Source: CAD feature listing. Evaluate the final solid. Frame: model axes, mm. A direction names the side the tool comes from. Give positions to 0.01 mm unless a question says otherwise; leave off trailing zeros. Order: outer loops, then holes, each group sorted by start corner. A loop starts at its lowest first (then second) coordinate and runs counter-clockwise, first axis right, second up.
from build123d import *

# Parameters (mm, degrees)
SKETCH_W      = 15.4
SKETCH_H      = 61
PAD_DEPTH     = 3
FILLET_R      = 4
PAD001_DEPTH  = 5
PAD002_DEPTH  = 5
SKETCH003_W   = 15.4
SKETCH003_H   = 6
PAD003_DEPTH  = 49
FILLET001_R   = 2.2
FILLET002_R   = 20
FILLET003_R   = 2.2
SKETCH004_W   = 4
SKETCH004_H   = 17
SKETCH004_W_2 = 2
SKETCH004_H_2 = 11
SKETCH004_W_3 = 2.5
SKETCH004_H_3 = 21
POCKET_DEPTH  = 54.801


with BuildPart() as part:
    # Sketch → Pad (new body)
    with BuildSketch(Plane.XZ):
        Rectangle(SKETCH_W, SKETCH_H)
    extrude(amount=PAD_DEPTH)

    # Fillet
    fillet_edges = [part.edges().sort_by_distance(p)[0] for p in [
        (7.7, -1.5, 30.5),
        (-7.7, -1.5, 30.5),
        (7.7, -1.5, -30.5),
        (-7.7, -1.5, -30.5),
    ]]
    fillet(fillet_edges, radius=FILLET_R)

    # Sketch001 (on Face2 of Fillet) → Pad001 (join)
    with BuildSketch(Plane(origin=(0, 0, 0), x_dir=(1, 0, 0), z_dir=(0, 1, 0))):
        with BuildLine():
            Line((-2.2, 16.65), (-2.2, 14.55))
            ThreePointArc((-2.2, 14.55), (0, 12.35), (2.2, 14.55))
            Line((2.2, 16.65), (2.2, 14.55))
            ThreePointArc((2.2, 16.65), (0, 18.85), (-2.2, 16.65))
        make_face()
        with BuildLine():
            Line((-2.2, -14.55), (-2.2, -16.65))
            ThreePointArc((-2.2, -16.65), (0, -18.85), (2.2, -16.65))
            Line((2.2, -14.55), (2.2, -16.65))
            ThreePointArc((2.2, -14.55), (0, -12.35), (-2.2, -14.55))
        make_face()
    extrude(amount=PAD001_DEPTH)

    # Sketch002 (on Face19 of Pad001) → Pad002 (join)
    with BuildSketch(Plane(origin=(0, 5, 0), x_dir=(1, 0, 0), z_dir=(0, 1, 0))):
        with BuildLine():
            Line((-2.2, 23.15), (-2.2, 14.55))
            ThreePointArc((-2.2, 14.55), (0, 12.35), (2.2, 14.55))
            Line((2.2, 23.15), (2.2, 14.55))
            ThreePointArc((2.2, 23.15), (0, 25.35), (-2.2, 23.15))
        make_face()
        with BuildLine():
            Line((-2.2, -8.05), (-2.2, -16.65))
            ThreePointArc((-2.2, -16.65), (0, -18.85), (2.2, -16.65))
            Line((2.2, -8.05), (2.2, -16.65))
            ThreePointArc((2.2, -8.05), (0, -5.85), (-2.2, -8.05))
        make_face()
    extrude(amount=PAD002_DEPTH)

    # Sketch003 (on Face5 of Pad002) → Pad003 (join)
    with BuildSketch(Plane.XZ.offset(3)):
        with Locations((0, 21.3)):
            Rectangle(SKETCH003_W, SKETCH003_H)
    extrude(amount=PAD003_DEPTH)

    # Fillet001
    fillet001_edges = [part.edges().sort_by_distance(p)[0] for p in [
        (7.7, -52, 21.3),
        (-7.7, -52, 21.3),
    ]]
    fillet(fillet001_edges, radius=FILLET001_R)

    # Fillet002
    fillet002_edges = [part.edges().sort_by_distance(p)[0] for p in [
        (0, -3, 18.3),
    ]]
    fillet(fillet002_edges, radius=FILLET002_R)

    # Fillet003
    fillet003_edges = [part.edges().sort_by_distance(p)[0] for p in [
        (0, -3, 24.3),
    ]]
    fillet(fillet003_edges, radius=FILLET003_R)

    # Sketch004 (on Face2 of Fillet003) → Pocket (cut, through all)
    with BuildSketch(Plane(origin=(0, 0, 24.3), x_dir=(-1, 0, 0), z_dir=(0, 0, 1))):
        with Locations((2.7, 15.5)):
            Rectangle(SKETCH004_W, SKETCH004_H)
        with Locations((2.7, 36.5)):
            Rectangle(SKETCH004_W_2, SKETCH004_H_2)
        with Locations((-3.55, 24.5)):
            Rectangle(SKETCH004_W_3, SKETCH004_H_3)
    extrude(amount=-POCKET_DEPTH, mode=Mode.SUBTRACT)


solid = part.part
1) Section query B-B on z = 11.5. Output: boundary loops of the cut face in (x, y).
Checks:
outline: (-7.7, -7.97) - (-4.7, -7.97) - (-4.7, -7) - (-0.7, -7) - (-0.7, -7.97) - (7.7, -7.97) - (7.7, 0) - (-7.7, 0) - close; (-2.2, 5) - (2.2, 5) - (2.2, 10) - (-2.2, 10) - close
2) Pull-direction query (Z, two-part tool) for faces 4 (the face through (0, 5, 9)), 5 (the face through (-0.05, 4.93, -12.35)), 6 (the face through (0, -37, 18.3)), 7 (the face through (-3, -42, 21)); classes: +Z half, -Z half, draft (parallel to the pull), parting line (faces both ways), or undercut.
Checks:
face 4: undercut
face 5: undercut
face 6: -Z half
face 7: draft
3) Reachability of faces 1 (the face through (0, -3, 29)), 2 (the face through (2.2, 7, -18)), 3 (the face through (0.05, 2.46, 12.35)) from +Z, -Z, +X, -X, +Y, -Y: full face, straight path, thin tool, end or side. Return the list, or none.
Checks:
face 1: +Z, +X, -X, -Y
face 2: +Z, -Z, +X, +Y
face 3: none
4) Ray query, L1, parallel to X at y = -30, z = 23.5; L2, parallel to X at y = -35.5, z = 22; L3, parallel to Y at x = 2.75, z = 24. Return the intervals inside material, ascending.
Checks:
L1: x = -7.7 to 2.3, 4.8 to 7.7
L2: x = -7.7 to -3.7, -1.7 to 7.7
L3: y = -52 to -35, -14 to 0
5) Section query C-C on y = -34. Output: boundary loops of the cut face in (x, z), and give its area (3 significant figures).
Checks:
outline: (-7.7, 18.3) - (-3.7, 18.3) - (-3.7, 24.3) - (-7.7, 24.3) - close; (-1.7, 18.3) - (2.3, 18.3) - (2.3, 24.3) - (-1.7, 24.3) - close; (4.8, 18.3) - (7.7, 18.3) - (7.7, 24.3) - (4.8, 24.3) - close
area: 65.4 mm2
6) Section query D-D on x = 0.5. Output: boundary loops of the cut face in (y, z), and give its area (3 significant figures).
Checks:
outline: (-52, 18.3) - (-23, 18.3) arc R20 cw to (-3, -1.7) - (-3, -30.5) - (0, -30.5) - (0, -18.79) - (5, -18.79) - (5, -25.29) - (10, -25.29) - (10, -12.41) - (0, -12.41) - (0, 12.41) - (5, 12.41) - (5, 5.91) - (10, 5.91) - (10, 18.79) - (0, 18.79) - (0, 30.5) - (-3, 30.5) - (-3, 26.5) arc R2.2 cw to (-5.2, 24.3) - (-52, 24.3) - close
area: 757 mm2
7) Section query A-A on y = -41. Output: boundary loops of the cut face in (x, z).
Checks:
outline: (-7.7, 18.3) - (-3.7, 18.3) - (-3.7, 24.3) - (-7.7, 24.3) - close; (-1.7, 18.3) - (7.7, 18.3) - (7.7, 24.3) - (-1.7, 24.3) - close
8) First-contact query: pin 1 Ø5 at (x, y) = (0.5, 3.5) entering from +Z; pin 2 Ø3 at (x, z) = (-3.5, 22.5) entering from +Y; pin 3 Ø3 at (x, y) = (0.5, -25) entering from +Z; pin 4 Ø4 at (x, z) = (-3, 11) entering from +Y. Flat tips, straight axial feed; report the tip coordinate or a pass-through.
Checks:
pin 1: stops at z = 18.85
pin 2: stops at y = 0
pin 3: stops at z = 24.3
pin 4: stops at y = 10
